Here's how the part is built. I have some questions about the finished solid (model axes, mm). Face numbers are marked on the shaded views. A direction names the side the tool comes from. Round coordinates to 2 decimals unless told otherwise and drop trailing zeros. Write each loop counter-clockwise with the first axis right and the second up, starting at its lowest first coordinate (ties: lowest second). Pieces come first, ordered by that corner, then holes. Notation, with made-up numbers: (78.5, 74.5) -> (102.5, 74.5) arc R19 ccw to (102.5, 81.5) -> close; hole circle Ø10 at (-16.5, -37.75). An arc over 180 degrees is marked (long way). Put each result on its own line as item: value. Start each with the question number.
1) I want a section at C-C, the plane z = -1.75. List the corners of the cut face in (x, y) for me, then the cut area to 3 significant figures.
2) I want a section at D-D, the plane x = -28. List the corners of the cut face in (y, z) for me, then the cut area to 3 significant figures.
3) If I drill on line 1 along Z through (x, y) = (-1.9, -16.5); line 2 along X through (y, z) = (-13.25, -25), over which ranges is the centre line in solid material (lowest first)? Write a range as [from, to].
4) Which directions (+Z, -Z, +X, -X, +Y, -Y) give clear straight access to the entire face, cutting with the end or side of a thin tool? Please do the marked faces 1 and 2.
5) I want a section at B-B, the plane y = -16.5. List the corners of the cut face in (x, z) for me, then the cut area to 3 significant figures.
6) Will these pins go through, and if not, where does the flat tip stop? P1, Ø8, axis at x = -10, z = -12.5, coming from the -Y side; P2, Ø13.5, axis at y = -15.5, z = -20, coming from the -X side.
7) I want a section at A-A, the plane z = -15. List the corners of the cut face in (x, y) for me.
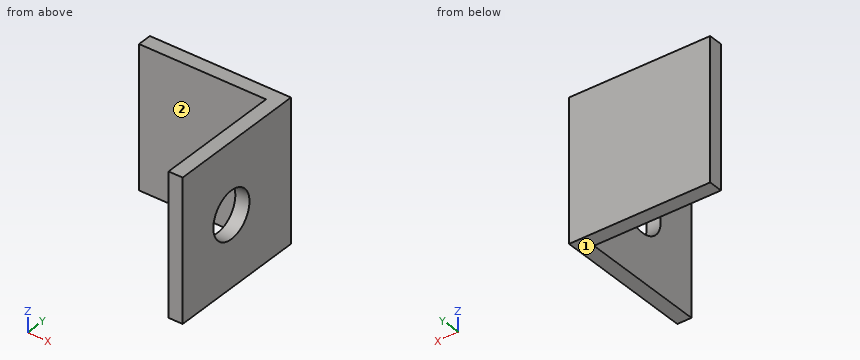
from build123d import *

# Parameters (mm, degrees)
BOSS_EXTRU_1_DEPTH = 30
D_GAGEMENT_M81_D   = 10
D_GAGEMENT_M82_D   = 10
D_GAGEMENT_M83_D   = 10
D_GAGEMENT_M84_D   = 10


with BuildPart() as part:
    # Esquisse1 → Boss.-Extru.1 (new body)
    with BuildSketch(Plane.XY):
        Polygon((0, 0), (0, -30), (-3, -30), (-3, -3), (-30, -3), (-30, 0), align=None)
    extrude(amount=-BOSS_EXTRU_1_DEPTH)

    # Dégagement M81 (through all)
    with Locations(Plane(origin=(-3, -21, 985), x_dir=(0, -1, 0), z_dir=(-1, 0, 0))):
        with Locations((-4.5, 1000), (-4.5, -1000)):
            Hole(D_GAGEMENT_M81_D / 2)

    # Dégagement M82 (through all)
    with Locations(Plane(origin=(33, -21, -1015), x_dir=(0, -1, 0), z_dir=(1, 0, 0))):
        with Locations((-4.5, 1000), (-4.5, -1000)):
            Hole(D_GAGEMENT_M82_D / 2)

    # Dégagement M83 (through all)
    with Locations(Plane(origin=(33, -21, 985), x_dir=(0, -1, 0), z_dir=(1, 0, 0))):
        with Locations((-4.5, 1000), (-4.5, -1000)):
            Hole(D_GAGEMENT_M83_D / 2)

    # Dégagement M84 (through all)
    with Locations(Plane(origin=(-3, -21, -1015), x_dir=(0, -1, 0), z_dir=(-1, 0, 0))):
        with Locations((-4.5, 1000), (-4.5, -1000)):
            Hole(D_GAGEMENT_M84_D / 2)


solid = part.part
Findings:
1. outline: (-30, -3) -> (-3, -3) -> (-3, -30) -> (0, -30) -> (0, 0) -> (-30, 0) -> close
1. area: 171 mm2
2. outline: (-3, -30) -> (0, -30) -> (0, 0) -> (-3, 0) -> close
2. area: 90.0 mm2
3. line 1: z = [-30, -20], [-10, 0]
3. line 2: x = [-3, 0]
4. face 1: -Z, +X, -X, +Y, -Y
4. face 2: +Z, -Z, -X, -Y
5. outline: (-3, -30) -> (0, -30) -> (0, -20) -> (-3, -20) -> close; (-3, -10) -> (0, -10) -> (0, 0) -> (-3, 0) -> close
5. area: 60.0 mm2
6. P1: stops at y = -3
6. P2: stops at x = -3
7. outline: (-30, -3) -> (-3, -3) -> (-3, -11.5) -> (0, -11.5) -> (0, 0) -> (-30, 0) -> close; (-3, -30) -> (0, -30) -> (0, -21.5) -> (-3, -21.5) -> close
